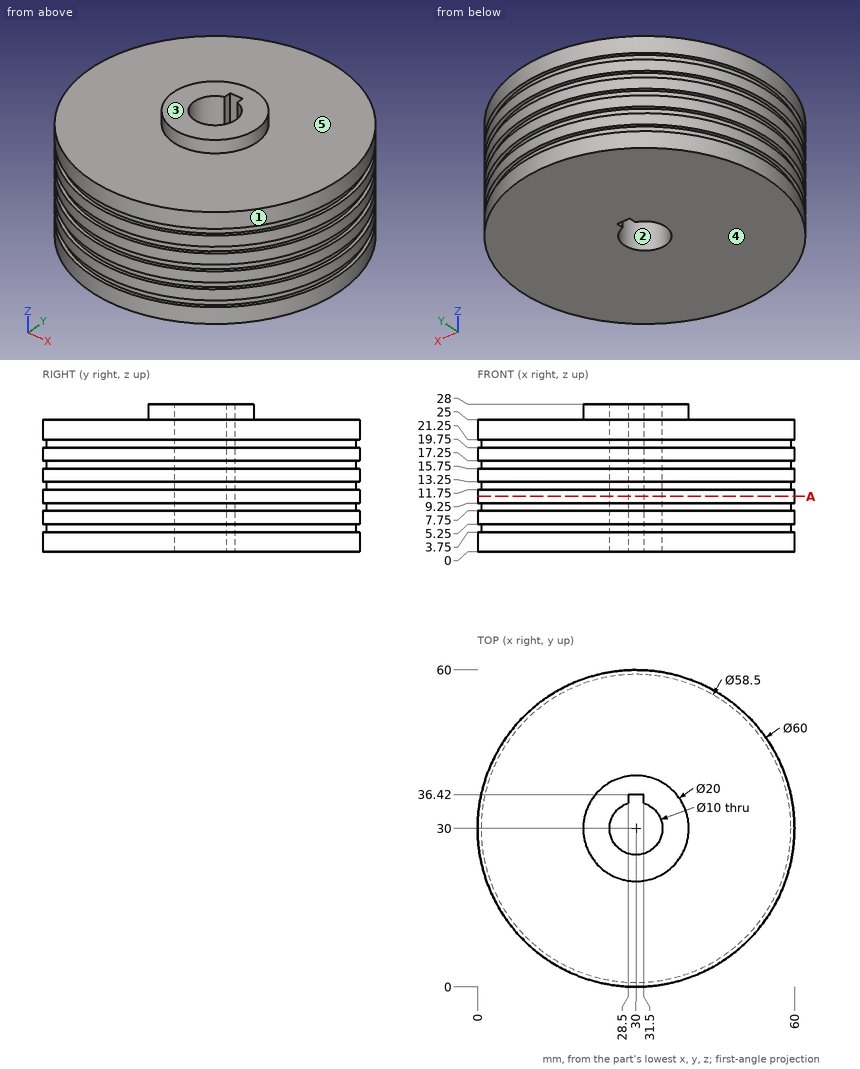
Study the drawing (mm; zero at the part's minimum x, y, z) and answer. A direction names the side the tool comes from. Give positions to 0.01 mm unless a question says otherwise; leave off trailing zeros. Write each loop counter-clockwise with the first axis right and the second up, starting at its lowest first coordinate (ties: lowest second). Pieces come first, ordered by that corner, then holes. Notation, with made-up numbers: (29, 35.5) - (78, 35.5) arc R21 cw to (78, 68.5) - close; hole circle Ø11 at (51.25, -8). An arc over 180 degrees is marked (long way). Write item = value, one per line. Start each with the question number.
Item 1: Find section A-A (z = 10.5). Give the vertices of the cut face in (x, y), then the cut area to 3 significant figures.
Item 2: Find the intervals of material crossed by probe 1 along X at (y, z) = (30, 21.5); probe 2 along Z at (x, y) = (26, 42.5); probe 3 along X at (y, z) = (29.5, 13) (1 decimal), in increasing order. Write a range as [from, to].
Item 3: A tool of negligible diameter and unlimited length cuts with its end or side. For the marked faces 4 and 5, from which of +Z, -Z, +X, -X, +Y, -Y can it reach the whole face along a straight path? Write none if from no direction.
Item 4: The mould has two halves that part along X. Classify the marked faces 1, 2 and 3: +X half, -X half, draft (parallel to the pull), parting line (faces both ways), or undercut.
Item 5: Each of these flat-tipped pins is pushed along its axis until it touches: P1, Ø3, axis at x = 34, z = 21, coming from the +Y side; P2, Ø3, axis at y = 45.5, z = 20.5, coming from the -X side; P3, Ø12, axis at y = 20, z = 11.5, coming from the -X side. Where does it stop, or does it pass through?
Response:
q1.outline = circle Ø60 at (30, 30); hole (28.5, 34.77) arc R5 ccw (long way) to (31.5, 34.77) - (31.5, 36.42) - (28.5, 36.42) - close
q1.area = 2,740 mm²
q2.probe_1 = [0, 25], [35, 60]
q2.probe_2 = [0, 25]
q2.probe_3 = [0.8, 25], [35, 59.2]
q3.face_4 = -Z, +X, -X, +Y, -Y
q3.face_5 = +Z
q4.face_1 = parting line
q4.face_2 = undercut
q4.face_3 = draft
q5.P1 = 59.89
q5.P2 = 3.57
q5.P3 = 0.27
